Print and shaded views of the part. All mm, measured from the part's lowest x, y and z. Coordinates: 2 decimals unless noted, no trailing zeros. Order: outer loops, then holes, each group sorted by start corner. A loop starts at its lowest first (then second) coordinate and runs counter-clockwise, first axis right, second up. Notation, with made-up numbers: (14, 31.5) -> (30, 31.5) arc R27 ccw to (30, 59.5) -> close; hole circle Ø10 at (-7.75, 22.5). An arc over 180 degrees is marked (long way). Write item = value, one per line. Start each with the question number.
Q1. Wall check: line 1 (X direction, y = 2.15, z = 3); line 2 (X direction, y = 2.35, z = 14); line 3 (Y direction, x = 10, z = 6.75). Give the ranges that are in metal, low to high. Write a range as from..to.
Q2. Cut at A-A, the plane y = 4. List the corners of the cut face in (x, z) (1 decimal).
Q3. Mould opens along X. For the marked faces 1, 2 and 3 say: +X half, -X half, draft (parallel to the pull), parting line (faces both ways), or undercut.
Q4. Cut at B-B, the plane z = 5. List the corners of the cut face in (x, y).
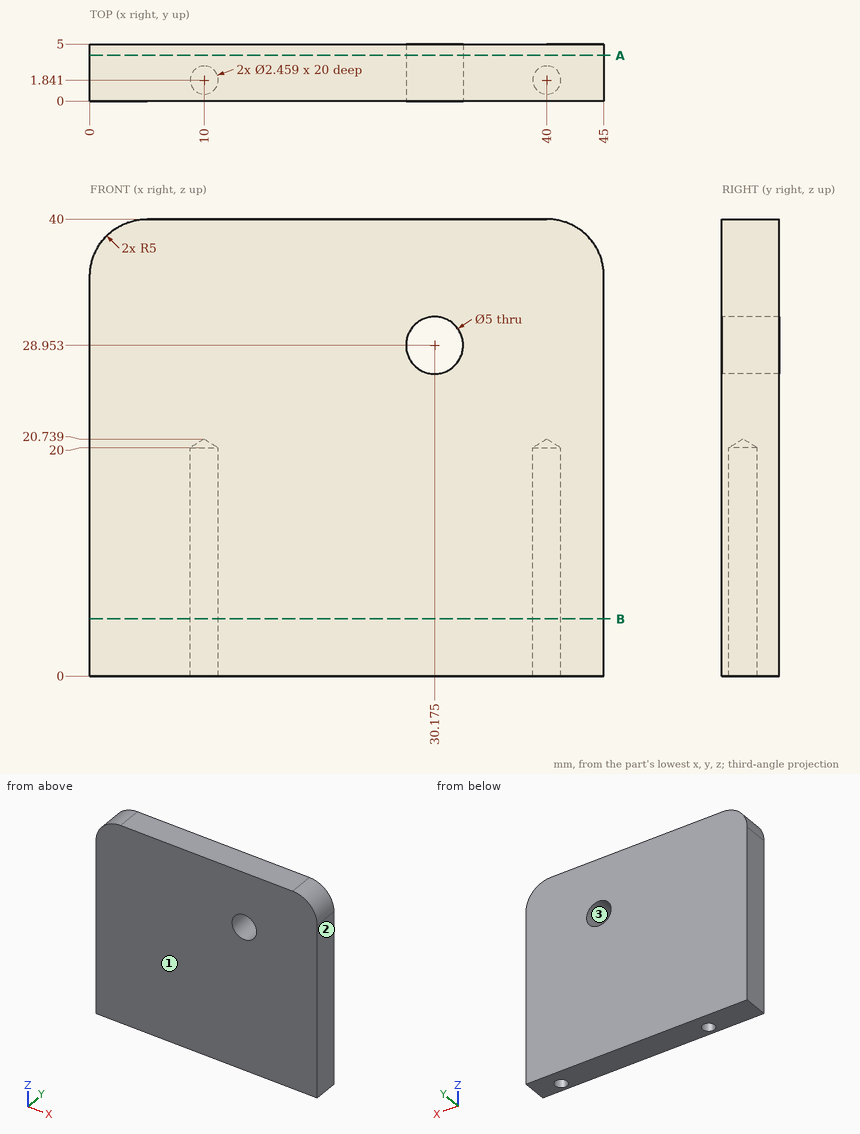
Here are the results:
q1.line_1 = 0..8.81, 11.19..38.81, 41.19..45
q1.line_2 = 0..8.88, 11.12..38.88, 41.12..45
q1.line_3 = 0..0.61, 3.07..5
q2.outline = (0, 0) -> (45, 0) -> (45, 35) arc R5 ccw to (40, 40) -> (5, 40) arc R5 ccw to (0, 35) -> close; hole circle Ø5 at (30.2, 29)
q3.face_1 = draft
q3.face_2 = +X half
q3.face_3 = undercut
q4.outline = (0, 0) -> (45, 0) -> (45, 5) -> (0, 5) -> close; hole circle Ø2.46 at (10, 1.84); hole circle Ø2.46 at (40, 1.84)
